Can you work these out from the model? Positions are in its coordinate system, mm. Give positions to 0.01 mm unless a question says otherwise; leave off trailing zeros. Order: outer loops, then holes, each group sorted by start corner. A loop starts at its lowest first (then second) coordinate and runs counter-clockwise, first axis right, second up. Notation, with made-up numbers: M -10,-37.75 L -4,-37.75 A14 ccw -4,-13.75 Z; hole C 21.25,-28 d7. An arc over 180 degrees is marked long. Use one line per item in the form item = value. Start each with the question number.
1. I want a section at B-B, the plane z = 0.35. List the corners of the cut face in (x, y) for me, and give its area (3 significant figures).
2. We'd pull the mould along Y, two halves only. Please class faces 1 (the face through (0.4, 8, 0.5)), 2 (the face through (-2, 0, 1)), 3 (the face through (-3.88, 3.21, 0.49)), 4 (the face through (1.25, 0.14, 0.49)): +Y half, -Y half, draft (parallel to the pull), parting line (faces both ways), or undercut.
3. I want a section at D-D, the plane y = 0. List the corners of the cut face in (x, z) for me.
4. I want a section at C-C, the plane x = -5. List the corners of the cut face in (y, z) for me.
5. I want a section at A-A, the plane x = -3.5. List the corners of the cut face in (y, z) for me, and give its area (3 significant figures).
6. I need wall thicknesses on L1, parallel to Y at x = -3.5, z = 0.7; L2, parallel to X at y = -4.5, z = 0.1; L3, parallel to X at y = 5, z = 0.1. Which ranges of each line are inside material? Lowest first, please.
```python
from build123d import *

# Parameters (mm, degrees)
SKETCH1_R           = 1.75
BOSS_EXTRUDE1_DEPTH = 1
CHAMFER1_SIZE       = 1


with BuildPart() as part:
    # Sketch1 → Boss-Extrude1 (new body)
    with BuildSketch(Plane.XY):
        with BuildLine():
            Line((7.5, -6.25), (7.5, -8))
            Line((7.5, -8), (-7.5, -8))
            Line((-7.5, -8), (-7.5, 8))
            Line((-7.5, 8), (7.5, 8))
            Line((7.5, 8), (7.5, 6.25))
            ThreePointArc((7.5, 6.25), (1.25, 0), (7.5, -6.25))
        make_face()
        with Locations((-3.5, 4.920147805)):
            Circle(SKETCH1_R, mode=Mode.SUBTRACT)
        with Locations((-3.5, -5.069977671)):
            Circle(SKETCH1_R, mode=Mode.SUBTRACT)
    extrude(amount=BOSS_EXTRUDE1_DEPTH)

    # Chamfer1
    chamfer1_edges = [part.edges().sort_by_distance(p)[0] for p in [
        (-7.5, -8, 0.5),
        (-7.5, 8, 0.5),
    ]]
    chamfer(chamfer1_edges, length=CHAMFER1_SIZE)


solid = part.part
```
Check result:
q1.outline = M -7.5,-7 L -6.5,-8 L 7.5,-8 L 7.5,-6.25 A6.25 cw 7.5,6.25 L 7.5,8 L -6.5,8 L -7.5,7 Z; hole C -3.5,-5.07 d3.5; hole C -3.5,4.92 d3.5
q1.area = 158 mm2
q2.face_1 = +Y half
q2.face_2 = draft
q2.face_3 = undercut
q2.face_4 = undercut
q3.outline = M -7.5,0 L 1.25,0 L 1.25,1 L -7.5,1 Z
q4.outline = M -8,0 L -5.97,0 L -5.97,1 L -8,1 Z; M -4.17,0 L 4.02,0 L 4.02,1 L -4.17,1 Z; M 5.82,0 L 8,0 L 8,1 L 5.82,1 Z
q5.outline = M -8,0 L -6.82,0 L -6.82,1 L -8,1 Z; M -3.32,0 L 3.17,0 L 3.17,1 L -3.32,1 Z; M 6.67,0 L 8,0 L 8,1 L 6.67,1 Z
q5.area = 9.00 mm2
q6.L1 = -8 to -6.82, -3.32 to 3.17, 6.67 to 8
q6.L2 = -7.5 to -5.15, -1.85 to 3.16
q6.L3 = -7.5 to -5.25, -1.75 to 3.75
